from build123d import *

# Parameters (mm, degrees)
SKIZZE1_W                              = 30
SKIZZE1_H                              = 25
AUFSATZ_LINEAR_AUSTRAGEN1_DEPTH        = 5
SKIZZE2_W                              = 5
SKIZZE2_H                              = 25
SCHNITT_LINEAR_AUSTRAGEN1_DEPTH        = 2.5
F_12_5_12_5_DURCHMESSER_BOHRUNG1_D     = 12.5
F_12_5_12_5_DURCHMESSER_BOHRUNG1_DEPTH = 5
F_12_5_12_5_DURCHMESSER_BOHRUNG1_TIP   = 3.755378869
DURCHGANGSLOCH_F_R_M31_D               = 3.2
DURCHGANGSLOCH_F_R_M31_DEPTH           = 5
DURCHGANGSLOCH_F_R_M31_TIP             = 0.96137699
SCHNITT_LINEAR_AUSTRAGEN2_DEPTH        = 33.882366095
SKIZZE8_W                              = 4.823257392
SKIZZE8_H                              = 2
SCHNITT_LINEAR_AUSTRAGEN3_DEPTH        = 10
VERRUNDUNG1_R                          = 10
M3_GEWINDEBOHRUNG2_D                   = 2.5


with BuildPart() as part:
    # Skizze1 → Aufsatz-Linear austragen1 (new body)
    with BuildSketch(Plane(origin=(0, 0, 0), x_dir=(1, 0, 0), z_dir=(0, 1, 0))):
        with Locations((15, 0)):
            Rectangle(SKIZZE1_W, SKIZZE1_H)
    extrude(amount=AUFSATZ_LINEAR_AUSTRAGEN1_DEPTH)

    # Skizze2 → Schnitt-Linear austragen1 (cut)
    with BuildSketch(Plane(origin=(0, 5, 0), x_dir=(1, 0, 0), z_dir=(0, 1, 0))):
        with Locations((2.5, 0)):
            Rectangle(SKIZZE2_W, SKIZZE2_H)
    extrude(amount=-SCHNITT_LINEAR_AUSTRAGEN1_DEPTH, mode=Mode.SUBTRACT)

    # Ø12.5 (12.5) Durchmesser Bohrung1
    with Locations(Plane(origin=(0, 5, 0), x_dir=(1, 0, 0), z_dir=(0, 1, 0))):
        with Locations((19, 0)):
            Hole(F_12_5_12_5_DURCHMESSER_BOHRUNG1_D / 2, depth=F_12_5_12_5_DURCHMESSER_BOHRUNG1_DEPTH)
            with Locations((0, 0, -(F_12_5_12_5_DURCHMESSER_BOHRUNG1_DEPTH + F_12_5_12_5_DURCHMESSER_BOHRUNG1_TIP / 2))):  # 118° drill point
                Cone(0, F_12_5_12_5_DURCHMESSER_BOHRUNG1_D / 2, F_12_5_12_5_DURCHMESSER_BOHRUNG1_TIP, mode=Mode.SUBTRACT)

    # Durchgangsloch für M31
    with Locations(Plane(origin=(0, 0, 0), x_dir=(-1, 0, 0), z_dir=(0, -1, 0))):
        with Locations((-2.5, 8), (-2.5, -8)):
            Hole(DURCHGANGSLOCH_F_R_M31_D / 2, depth=DURCHGANGSLOCH_F_R_M31_DEPTH)
            with Locations((0, 0, -(DURCHGANGSLOCH_F_R_M31_DEPTH + DURCHGANGSLOCH_F_R_M31_TIP / 2))):  # 118° drill point
                Cone(0, DURCHGANGSLOCH_F_R_M31_D / 2, DURCHGANGSLOCH_F_R_M31_TIP, mode=Mode.SUBTRACT)

    # Skizze7 → Schnitt-Linear austragen2 (cut, through all)
    with BuildSketch(Plane(origin=(0, 5, 0), x_dir=(1, 0, 0), z_dir=(0, 1, 0))):
        Polygon((10, 12.5), (14.330127019, 10), (30, 10), (30, 12.5), align=None)
        Polygon((30, -10), (14.330127019, -10), (10, -12.5), (30, -12.5), align=None)
    extrude(amount=-SCHNITT_LINEAR_AUSTRAGEN2_DEPTH, mode=Mode.SUBTRACT)

    # Skizze8 → Schnitt-Linear austragen3 (cut)
    with BuildSketch(Plane(origin=(0, 5, 0), x_dir=(1, 0, 0), z_dir=(0, 1, 0))):
        with Locations((27.588371304, 0)):
            Rectangle(SKIZZE8_W, SKIZZE8_H)
    extrude(amount=-SCHNITT_LINEAR_AUSTRAGEN3_DEPTH, mode=Mode.SUBTRACT)

    # Verrundung1
    verrundung1_edges = [part.edges().sort_by_distance(p)[0] for p in [
        (14.330127019, 2.5, -10),
        (14.330127019, 2.5, 10),
    ]]
    fillet(verrundung1_edges, radius=VERRUNDUNG1_R)

    # M3 Gewindebohrung2 (through all)
    with Locations(Plane.XY.offset(10)):
        with Locations((19, 2.5)):
            Hole(M3_GEWINDEBOHRUNG2_D / 2)


solid = part.part
Input: part model. Units: mm. Frame: model coordinates. A direction names the side the tool comes from. Coordinates: 2 decimals unless noted, no trailing zeros. Loops run counter-clockwise (first coordinate to the right, second up) from the corner with the lowest first, then second, coordinate; pieces in that order, holes last. Notation, with made-up numbers: (78.25, 45.5) -> (83.25, 45.5) arc R34 cw to (83.25, 80.5) -> close; hole circle Ø9 at (-17.5, 68). An arc over 180 degrees is marked (long way). Write item = value, one per line. Start each with the question number.
Item 1: Cut plane A-A, the plane x = 27. Return loops of the section in (y, z).
Item 2: Cut plane B-B, the plane x = 19. Return loops of the section in (y, z).
Item 3: First-contact query: P1, Ø1.4, axis at x = 27.5, y = 2.5, coming from the -Z side; P2, Ø1.5, axis at x = 21, y = 2, coming from the +Z side; P3, Ø0.8, axis at y = 4, z = 6, coming from the -X side. Flat tips, straight axial feed; report the tip coordinate or a pass-through.
Item 4: Cut plane D-D, the plane x = 2.5. Return loops of the section in (y, z).
Item 5: Reachability of faces 1 (the face through (28, 3, 1)), 2 (the face through (24, 3, 10)), 3 (the face through (12, 5, 0)), 4 (the face through (12.755, 2.465, 0.261)), 5 (the face through (23, 3, -10)) from +Z, -Z, +X, -X, +Y, -Y: full face, straight path, thin tool, end or side. Return the list, or none.
Item 6: Mould query, pull axis Z, two halves, no side actions, for faces 6 (the face through (10.99, 2.54, -11.93)), 7 (the face through (28, 3, -1)), 8 (the face through (5, 4, 0)), 9 (the face through (2.15, 1.27, 9.56)). Classes: pulls with the +Z half, pulls with the -Z half, needs draft (parallel to the pull), parting line crosses it, or undercut.
Item 7: Material intervals for line 1 (Z direction, x = 2.5, y = 1.15); line 2 (X direction, y = 1.85, z = 8); line 3 (Y direction, x = 19, z = 8.65), sorted ascending.
Item 8: Cut plane C-C, the plane y = 1.65. Return loops of the section in (x, z), plus the area to 3 significant figures.
Ans:
q1.outline = (0, -10) -> (5, -10) -> (5, -1) -> (0, -1) -> close; (0, 1) -> (5, 1) -> (5, 10) -> (0, 10) -> close
q2.outline = (0, -10) -> (1.25, -10) -> (1.25, -6.25) -> (0, -6.25) -> close; (0, 6.25) -> (1.25, 6.25) -> (1.25, 10) -> (0, 10) -> close; (3.75, -10) -> (5, -10) -> (5, -6.25) -> (3.75, -6.25) -> close; (3.75, 6.25) -> (5, 6.25) -> (5, 10) -> (3.75, 10) -> close
q3.P1 = -10
q3.P2 = 10
q3.P3 = 5
q4.outline = (0, -12.5) -> (2.5, -12.5) -> (2.5, -9.6) -> (0, -9.6) -> close; (0, -6.4) -> (2.5, -6.4) -> (2.5, 6.4) -> (0, 6.4) -> close; (0, 9.6) -> (2.5, 9.6) -> (2.5, 12.5) -> (0, 12.5) -> close
q5.face_1 = +X, +Y, -Y
q5.face_2 = +Z, +X, +Y, -Y
q5.face_3 = +Z, -Z, +X, -X, +Y
q5.face_4 = +Y, -Y
q5.face_5 = -Z, +X, +Y, -Y
q6.face_6 = pulls with the -Z half
q6.face_7 = undercut
q6.face_8 = needs draft
q6.face_9 = undercut
q7.line_1 = -12.5 to -9.6, -6.4 to 6.4, 9.6 to 12.5
q7.line_2 = 0 to 0.9, 4.1 to 17.93, 20.07 to 30
q7.line_3 = 0 to 1.25, 3.75 to 5
q8.outline = (0, -12.5) -> (10, -12.5) -> (12.01, -11.34) arc R10 cw to (17.01, -10) -> (18.08, -10) -> (18.08, -6.18) arc R6.25 cw to (18.08, 6.18) -> (18.08, 10) -> (17.01, 10) arc R10 cw to (12.01, 11.34) -> (10, 12.5) -> (0, 12.5) -> close; (19.92, -10) -> (30, -10) -> (30, -1) -> (25.18, -1) -> (25.18, -0.95) arc R6.25 cw to (19.92, -6.18) -> close; (19.92, 6.18) arc R6.25 cw to (25.18, 0.95) -> (25.18, 1) -> (30, 1) -> (30, 10) -> (19.92, 10) -> close; hole circle Ø3.2 at (2.5, -8); hole circle Ø3.2 at (2.5, 8)
q8.area = 500 mm²
